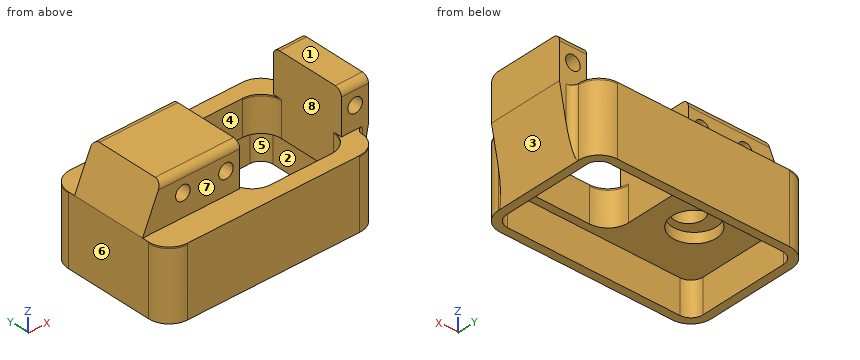
```python
from build123d import *

# Parameters (mm, degrees)
SKETCH2_W           = 62.8
SKETCH2_H           = 38.3
SKETCH2_R           = 4.25
SKETCH2_W_2         = 30
SKETCH2_H_2         = 29
BOSS_EXTRUDE1_DEPTH = 10
SKETCH2_3_W         = 62.8
SKETCH2_3_H         = 38.3
SKETCH2_3_W_2       = 58
SKETCH2_3_H_2       = 33.5
BOSS_EXTRUDE2_DEPTH = 10
SKETCH2_4_R         = 6.5
CUT_EXTRUDE1_DEPTH  = 3
FILLET1_R           = 3.6
FILLET2_R           = 6
BOSS_EXTRUDE3_START = 0.4
SKETCH4_R           = 4.25
BOSS_EXTRUDE3_DEPTH = 0.4
SKETCH5_W           = 23.1
SKETCH5_H           = 22.25
SKETCH5_W_2         = 8
BOSS_EXTRUDE4_DEPTH = 12.6
SKETCH6_R           = 2.15
CUT_EXTRUDE2_DEPTH  = 22.25
BOSS_EXTRUDE6_DEPTH = 22.25
FILLET5_R           = 2
FILLET6_R           = 2
SKETCH4_2_R         = 4.25
CUT_EXTRUDE3_DEPTH  = 5
FILLET7_R           = 1


with BuildPart() as part:
    # Sketch2 → Boss-Extrude1 (new body)
    with BuildSketch(Plane.XY):
        with Locations((29, -16.75)):
            Rectangle(SKETCH2_W, SKETCH2_H)
        with Locations((16.2, -16.75)):
            Circle(SKETCH2_R, mode=Mode.SUBTRACT)
        with Locations((41.25, -16.75)):
            Rectangle(SKETCH2_W_2, SKETCH2_H_2, mode=Mode.SUBTRACT)
    extrude(amount=BOSS_EXTRUDE1_DEPTH)

    # Sketch2<3> → Boss-Extrude2 (add)
    with BuildSketch(Plane.XY):
        with Locations((29, -16.75)):
            Rectangle(SKETCH2_3_W, SKETCH2_3_H)
        with Locations((29, -16.75)):
            Rectangle(SKETCH2_3_W_2, SKETCH2_3_H_2, mode=Mode.SUBTRACT)
    extrude(amount=-BOSS_EXTRUDE2_DEPTH)

    # Sketch2<4> → Cut-Extrude1 (cut)
    with BuildSketch(Plane.XY):
        with Locations((14.45, -16.75)):
            Circle(SKETCH2_4_R)
    extrude(amount=CUT_EXTRUDE1_DEPTH, mode=Mode.SUBTRACT)

    # Fillet1
    fillet1_edges = [part.edges().sort_by_distance(p)[0] for p in [
        (58, 0, -5),
        (0, 0, -5),
        (0, -33.5, -5),
        (58, -33.5, -5),
    ]]
    fillet(fillet1_edges, radius=FILLET1_R)

    # Fillet2
    fillet2_edges = [part.edges().sort_by_distance(p)[0] for p in [
        (26.25, -2.25, 5),
        (26.25, -31.25, 5),
        (56.25, -31.25, 5),
        (56.25, -2.25, 5),
        (60.4, -35.9, 0),
        (-2.4, -35.9, 0),
        (-2.4, 2.4, 0),
        (60.4, 2.4, 0),
    ]]
    fillet(fillet2_edges, radius=FILLET2_R)

    # Sketch4 → Boss-Extrude3 (add)
    with BuildSketch(Plane.XY.offset(10).offset(BOSS_EXTRUDE3_START)):
        with BuildLine():
            Line((3.6, -35.9), (54.4, -35.9))
            ThreePointArc((54.4, -35.9), (58.642640687, -34.142640687), (60.4, -29.9))
            Line((60.4, -29.9), (60.4, -3.6))
            ThreePointArc((60.4, -3.6), (58.642640687, 0.642640687), (54.4, 2.4))
            Line((54.4, 2.4), (3.6, 2.4))
            ThreePointArc((3.6, 2.4), (-0.642640687, 0.642640687), (-2.4, -3.6))
            Line((-2.4, -3.6), (-2.4, -29.9))
            ThreePointArc((-2.4, -29.9), (-0.642640687, -34.142640687), (3.6, -35.9))
        make_face()
        with Locations((16.2, -16.75)):
            Circle(SKETCH4_R, mode=Mode.SUBTRACT)
        with BuildLine():
            Line((56.25, -8.25), (56.25, -25.25))
            ThreePointArc((56.25, -25.25), (54.492640687, -29.492640687), (50.25, -31.25))
            Line((50.25, -31.25), (32.25, -31.25))
            ThreePointArc((32.25, -31.25), (28.007359313, -29.492640687), (26.25, -25.25))
            Line((26.25, -25.25), (26.25, -8.25))
            ThreePointArc((26.25, -8.25), (28.007359313, -4.007359313), (32.25, -2.25))
            Line((32.25, -2.25), (50.25, -2.25))
            ThreePointArc((50.25, -2.25), (54.492640687, -4.007359313), (56.25, -8.25))
        make_face(mode=Mode.SUBTRACT)
    extrude(amount=-BOSS_EXTRUDE3_DEPTH)

    # Sketch5 → Boss-Extrude4 (add)
    with BuildSketch(Plane.XY.offset(10.4)):
        with Locations((14.7, -16.75)):
            Rectangle(SKETCH5_W, SKETCH5_H)
        with Locations((60.25, -16.75)):
            Rectangle(SKETCH5_W_2, SKETCH5_H)
    extrude(amount=BOSS_EXTRUDE4_DEPTH)

    # Sketch6 → Cut-Extrude2 (cut)
    with BuildSketch(Plane(origin=(0, -5.625, 0), x_dir=(1, 0, 0), z_dir=(0, 1, 0))):
        with Locations(Location((9.5, -16.95, 0), (0, 0, 270))):
            Circle(SKETCH6_R)
        with Locations(Location((22.2, -16.95, 0), (0, 0, 270))):
            Circle(SKETCH6_R)
        with Locations(Location((60.3, -16.95, 0), (0, 0, 270))):
            Circle(SKETCH6_R)
    extrude(amount=-CUT_EXTRUDE2_DEPTH, mode=Mode.SUBTRACT)

    # Sketch7 → Boss-Extrude6 (add)
    with BuildSketch(Plane(origin=(0, -5.625, 0), x_dir=(1, 0, 0), z_dir=(0, 1, 0))):
        Polygon((-2.4, -10.4), (3.15, -23), (3.15, -10.4), align=None)
        Polygon((60.4, -10.4), (64.25, -10.4), (60.4, 10), align=None)
    extrude(amount=-BOSS_EXTRUDE6_DEPTH)

    # Fillet5
    fillet5_edges = [part.edges().sort_by_distance(p)[0] for p in [
        (60.4, -27.875, 0.2),
        (60.4, -5.625, 0.2),
    ]]
    fillet(fillet5_edges, radius=FILLET5_R)

    # Fillet6
    fillet6_edges = [part.edges().sort_by_distance(p)[0] for p in [
        (60.25, -5.625, 23),
        (60.25, -27.875, 23),
        (14.7, -5.625, 23),
        (14.7, -27.875, 23),
    ]]
    fillet(fillet6_edges, radius=FILLET6_R)

    # Sketch4<2> → Cut-Extrude3 (cut)
    with BuildSketch(Plane.XY.offset(10)):
        with Locations((16.2, -16.75)):
            Circle(SKETCH4_2_R)
    extrude(amount=CUT_EXTRUDE3_DEPTH, mode=Mode.SUBTRACT)

    # Fillet7
    fillet7_edges = [part.edges().sort_by_distance(p)[0] for p in [
        (11.95, -16.75, 15),
    ]]
    fillet(fillet7_edges, radius=FILLET7_R)


solid = part.part
```
The listing builds one solid part. Answer for the finished solid, in the listing's coordinates (mm). Face numbers are marked on the shaded views. A direction names the side the tool comes from. Coordinates: 2 decimals unless noted, no trailing zeros. Write each loop counter-clockwise with the first axis right and the second up, starting at its lowest first coordinate (ties: lowest second). Pieces come first, ordered by that corner, then holes. Notation, with made-up numbers: (4, -13) -> (63, -13) arc R9 ccw to (63, 2) -> close; hole circle Ø1 at (35, 40). An arc over 180 degrees is marked (long way). Write each question's results on one line, items separated by ' | '. Start each with the question number.
1) A tool of negligible diameter and unlimited length cuts with its end or side. For the marked faces 4, 5, 6, 7 and 8, from which of +Z, -Z, +X, -X, +Y, -Y can it reach the whole face along a straight path? Write none if from no direction.
2) A cutting plane is placed at C-C (x = 40.5). Determine the outline of the cut face in (y, z), then the cut area to 3 significant figures.
3) A cutting plane is placed at A-A (x = 22.2). Determine the outline of the cut face in (y, z) (3 decimals), then the cut area to 3 significant figures.
4) Flat-ended cylindrical pins translate along their axes: pin 1 Ø8.5 at (x, z) = (7, 15.5) entering from -Y (3 decimals); pin 2 Ø21 at (x, y) = (14.45, -16.75) entering from -Z; pin 3 Ø5 at (y, z) = (-15.5, -3) entering from +X; pin 4 Ø4 at (x, z) = (9.5, 16.95) entering from -Y. Find the tip coordinate at first contact, or state that the pin passes through.
5) Straight lines are drawn through the part: probe 1 along Y at (x, z) = (40.5, -4.5); probe 2 along Y at (x, z) = (16.2, 5.5); probe 3 along X at (y, z) = (-19, 16). For each, find the intervals that lie inside material, in ascending order.
6) A cutting plane is placed at B-B (z = 16.95). Determine the outline of the cut face in (x, y) (3 decimals).
7) A cutting plane is placed at D-D (y = -18). Count the separate pieces of the cut face and the enclosed holes in it, then the cut area to 3 significant figures.
8) For a pull along X with two mould halves and no side action, classify the marked faces 1, 2 and 3 as +X half, -X half, draft (parallel to the pull), parting line (faces both ways), or undercut.
Values follow:
1) face 4: +Z, -Z | face 5: -Z | face 6: +Z, -Z, -X, +Y, -Y | face 7: +Z, +X, -X, -Y | face 8: +Z
2) outline: (-35.9, -10) -> (-33.5, -10) -> (-33.5, 0) -> (-31.25, 0) -> (-31.25, 10.4) -> (-35.9, 10.4) -> close; (-2.25, 0) -> (0, 0) -> (0, -10) -> (2.4, -10) -> (2.4, 10.4) -> (-2.25, 10.4) -> close | area: 145 mm²
3) outline: (-35.9, -10) -> (-33.5, -10) -> (-33.5, 0) -> (0, 0) -> (0, -10) -> (2.4, -10) -> (2.4, 10.4) -> (-5.625, 10.4) -> (-5.625, 14.8) -> (-27.875, 14.8) -> (-27.875, 10.4) -> (-35.9, 10.4) -> close; (-27.875, 19.1) -> (-5.625, 19.1) -> (-5.625, 21) arc R2 ccw to (-7.625, 23) -> (-25.875, 23) arc R2 ccw to (-27.875, 21) -> close | area: 629 mm²
4) pin 1: y = -27.875 | pin 2: z = 0 | pin 3: x = 62.19 | pin 4: through
5) probe 1: -35.9 to -33.5, 0 to 2.4 | probe 2: -35.9 to -21, -12.5 to 2.4 | probe 3: 0.07 to 7.57, 11.43 to 20.27, 24.13 to 26.25, 56.25 to 58.37, 62.23 to 64.25
6) outline: (0.485, -27.875) -> (7.35, -27.875) -> (7.35, -5.625) -> (0.485, -5.625) -> close; (11.65, -27.875) -> (20.05, -27.875) -> (20.05, -5.625) -> (11.65, -5.625) -> close; (24.35, -27.875) -> (26.25, -27.875) -> (26.25, -5.625) -> (24.35, -5.625) -> close; (56.25, -27.875) -> (58.15, -27.875) -> (58.15, -5.625) -> (56.25, -5.625) -> close; (62.45, -27.875) -> (64.25, -27.875) -> (64.25, -5.625) -> (62.45, -5.625) -> close
7) separate pieces: 2 | enclosed holes: 3 | area: 676 mm²
8) face 1: draft | face 2: undercut | face 3: +X half
